Part model, mm, in its own coordinate system. A direction names the side the tool comes from. Round coordinates to 2 decimals unless told otherwise and drop trailing zeros. Loops run counter-clockwise (first coordinate to the right, second up) from the corner with the lowest first, then second, coordinate; pieces in that order, holes last. Notation, with made-up numbers: M 3,16.25 L 10,16.25 A20 ccw 10,40.25 Z; hole C -4,86 d7. An arc over 180 degrees is marked long. Write each question's results on one line, items separated by ' | '.
from build123d import *

# Parameters (mm, degrees)
CROQUIS1_W              = 140
CROQUIS1_H              = 45
CROQUIS1_W_2            = 136
CROQUIS1_H_2            = 41
SALIENTE_EXTRUIR1_DEPTH = 10
CROQUIS2_W              = 140
CROQUIS2_H              = 45
SALIENTE_EXTRUIR2_DEPTH = 2
CHAFL_N1_SIZE           = 1
CROQUIS3_W              = 9
CROQUIS3_H              = 12
CROQUIS3_R              = 1.75
SALIENTE_EXTRUIR3_DEPTH = 3.5
CHAFL_N2_SIZE           = 2
CROQUIS4_W              = 20
CROQUIS4_H              = 7.5
CORTAR_EXTRUIR1_DEPTH   = 3.5


with BuildPart() as part:
    # Croquis1 → Saliente-Extruir1 (new body)
    with BuildSketch(Plane(origin=(0, 0, 0), x_dir=(1, 0, 0), z_dir=(0, 1, 0))):
        Rectangle(CROQUIS1_W, CROQUIS1_H)
        Rectangle(CROQUIS1_W_2, CROQUIS1_H_2, mode=Mode.SUBTRACT)
    extrude(amount=SALIENTE_EXTRUIR1_DEPTH)

    # Croquis2 → Saliente-Extruir2 (add)
    with BuildSketch(Plane(origin=(0, 10, 0), x_dir=(1, 0, 0), z_dir=(0, 1, 0))):
        Rectangle(CROQUIS2_W, CROQUIS2_H)
    extrude(amount=-SALIENTE_EXTRUIR2_DEPTH)

    # Chaflán1
    chafl_n1_edges = [part.edges().sort_by_distance(p)[0] for p in [
        (-70, 10, 0),
        (0, 10, 22.5),
        (70, 10, 0),
        (70, 5, 22.5),
        (-70, 5, 22.5),
        (-70, 5, -22.5),
        (70, 5, -22.5),
        (0, 10, -22.5),
    ]]
    chamfer(chafl_n1_edges, length=CHAFL_N1_SIZE)

    # Croquis3 → Saliente-Extruir3 (add)
    with BuildSketch(Plane(origin=(0, 0, 0), x_dir=(1, 0, 0), z_dir=(0, 1, 0))):
        with Locations((-50, 28.5)):
            Rectangle(CROQUIS3_W, CROQUIS3_H)
        with Locations((-50, 30)):
            Circle(CROQUIS3_R, mode=Mode.SUBTRACT)
        with Locations((50, 28.5)):
            Rectangle(CROQUIS3_W, CROQUIS3_H)
        with Locations((50, 30)):
            Circle(CROQUIS3_R, mode=Mode.SUBTRACT)
        with Locations((-50, -28.5)):
            Rectangle(CROQUIS3_W, CROQUIS3_H)
        with Locations((-50, -30)):
            Circle(CROQUIS3_R, mode=Mode.SUBTRACT)
        with Locations((50, -28.5)):
            Rectangle(CROQUIS3_W, CROQUIS3_H)
        with Locations((50, -30)):
            Circle(CROQUIS3_R, mode=Mode.SUBTRACT)
    extrude(amount=SALIENTE_EXTRUIR3_DEPTH)

    # Chaflán2
    chafl_n2_edges = [part.edges().sort_by_distance(p)[0] for p in [
        (-50, 3.5, 22.5),
        (-54.5, 1.75, 22.5),
        (-54.5, 1.75, 34.5),
        (-45.5, 1.75, 34.5),
        (-45.5, 1.75, 22.5),
        (50, 3.5, 22.5),
        (45.5, 1.75, 22.5),
        (45.5, 1.75, 34.5),
        (54.5, 1.75, 34.5),
        (54.5, 1.75, 22.5),
        (-50, 3.5, -22.5),
        (-54.5, 1.75, -34.5),
        (-54.5, 1.75, -22.5),
        (-45.5, 1.75, -22.5),
        (-45.5, 1.75, -34.5),
        (50, 3.5, -22.5),
        (45.5, 1.75, -34.5),
        (45.5, 1.75, -22.5),
        (54.5, 1.75, -22.5),
        (54.5, 1.75, -34.5),
    ]]
    chamfer(chafl_n2_edges, length=CHAFL_N2_SIZE)

    # Croquis4 → Cortar-Extruir1 (cut)
    with BuildSketch(Plane.ZY.offset(70)):
        with Locations((0, 3.75)):
            Rectangle(CROQUIS4_W, CROQUIS4_H)
    extrude(amount=-CORTAR_EXTRUIR1_DEPTH, mode=Mode.SUBTRACT)


solid = part.part
Item 1: Band-saw the part on B-B on x = 50. Give the cut face in (y, z), and give its area (4 significant figures).
Filled sheet:
outline: M 0,-34.5 L 3.5,-34.5 L 3.5,-31.75 L 0,-31.75 Z; M 0,-28.25 L 3.5,-28.25 L 3.5,-24.5 L 5.5,-22.5 L 9,-22.5 L 10,-21.5 L 10,21.5 L 9,22.5 L 5.5,22.5 L 3.5,24.5 L 3.5,28.25 L 0,28.25 L 0,20.5 L 8,20.5 L 8,-20.5 L 0,-20.5 Z; M 0,31.75 L 3.5,31.75 L 3.5,34.5 L 0,34.5 Z | area: 184.5 mm^2
Item 2: Which spindle directions (+Z, -Z, +X, -X, +Y, -Y) get a long thin tool onto all of the face, cutting with end or side? Do faces 4 (the flat face through (54.5, 2, 29)), 5 (the flat face through (45.5, 2, -28)), 6 (the flat face through (-54.5, 2, -28)). Say none if no direction does.
Filled sheet:
face 4: +Z, +X, +Y, -Y | face 5: -Z, +Y, -Y | face 6: -Z, -X, +Y, -Y
Item 3: Band-saw the part on D-D on z = -19. Give the cut face in (x, y), and give its area (3 significant figures).
Filled sheet:
outline: M -70,0 L -68,0 L -68,8 L 68,8 L 68,0 L 70,0 L 70,9 L 69,10 L -69,10 L -70,9 Z | area: 311 mm^2
Item 4: Wall check: L1, parallel to X at y = 2.05, z = -30; L2, parallel to Z at x = -50, y = 1.5; L3, parallel to Z at x = 1, y = 2.5. Give the ranges that are in metal, low to high.
Filled sheet:
L1: -54.5 to -51.75, -48.25 to -45.5, 45.5 to 48.25, 51.75 to 54.5 | L2: -34.5 to -31.75, -28.25 to -20.5, 20.5 to 28.25, 31.75 to 34.5 | L3: -22.5 to -20.5, 20.5 to 22.5
Item 5: Band-saw the part on C-C on x = -40. Give the cut face in (y, z).
Filled sheet:
outline: M 0,-22.5 L 9,-22.5 L 10,-21.5 L 10,21.5 L 9,22.5 L 0,22.5 L 0,20.5 L 8,20.5 L 8,-20.5 L 0,-20.5 Z
Item 6: Drop flat-ended pins along their axis: P1, Ø6, axis at x = -6.5, y = 8.5, coming from the -Z side; P2, Ø2.5, axis at x = -48, z = 29, coming from the +Y side; P3, Ø2, axis at x = -69.5, y = 2, coming from the +Z side. Give the stop position or say it passes through.
Filled sheet:
P1: z = -22.5 | P2: y = 3.5 | P3: z = 22.5
Item 7: Band-saw the part on A-A on z = 30. Give the cut face in (x, y).
Filled sheet:
outline: M -54.5,0 L -51.75,0 L -51.75,3.5 L -54.5,3.5 Z; M -48.25,0 L -45.5,0 L -45.5,3.5 L -48.25,3.5 Z; M 45.5,0 L 48.25,0 L 48.25,3.5 L 45.5,3.5 Z; M 51.75,0 L 54.5,0 L 54.5,3.5 L 51.75,3.5 Z
Item 8: Two-plate mould, pull along Z, no slides. Class faces 1 (the flat face through (-1, 4, 22.5)), 2 (the cylindrical face through (-48.383, 1.726, -29.33)), 3 (the flat face through (54.5, 2, -28)): +Z half, -Z half, draft (parallel to the pull), parting line (faces both ways), or undercut.
Filled sheet:
face 1: +Z half | face 2: undercut | face 3: draft
